```python
from build123d import *

# Parameters (mm, degrees)
EXTRUDE_1_DEPTH     = 20
SKETCH_2_R          = 4
CUT_EXTRUDE_1_DEPTH = 20


with BuildPart() as part:
    # 草图1 → 凸台-拉伸1 (new body)
    with BuildSketch(Plane.XY):
        with BuildLine():
            Line((0, -15), (350, -15))
            ThreePointArc((350, -15), (365, 0), (350, 15))
            Line((350, 15), (0, 15))
            ThreePointArc((0, 15), (-15, 0), (0, -15))
        make_face()
    extrude(amount=EXTRUDE_1_DEPTH)

    # 草图2 → 切除-拉伸1 (cut)
    with BuildSketch(Plane.XY):
        Circle(SKETCH_2_R)
        with Locations((350, 0)):
            Circle(SKETCH_2_R)
    extrude(amount=CUT_EXTRUDE_1_DEPTH, mode=Mode.SUBTRACT)


solid = part.part
```
Verification items for the finished model (mm, model axes). Round coordinates to 2 decimals unless told otherwise and drop trailing zeros. Write each loop counter-clockwise with the first axis right and the second up, starting at its lowest first coordinate (ties: lowest second). Pieces come first, ordered by that corner, then holes. Notation, with made-up numbers: (12.5, 76) -> (29.5, 76) arc R13 ccw to (29.5, 94) -> close; hole circle Ø8 at (52, -13.75). An arc over 180 degrees is marked (long way). Write each question's results on one line, items separated by ' | '. Start each with the question number.
1. Depth check by flat-ended pin: P1, Ø8, axis at y = -9, z = 17, coming from the +X side; P2, Ø1, axis at y = -8, z = 5.5, coming from the -X side; P3, Ø8, axis at y = 10, z = 6.5, coming from the +X side; P4, Ø10, axis at x = 308, y = -10.5, coming from the -Z side. Enter the tip coordinate at first touch or a pass-through.
2. Material ranges on probe 1 along Y at (x, z) = (0, 7.75); probe 2 along X at (y, z) = (13, 16); probe 3 along X at (y, z) = (6, 15), recorded low to high. Write a range as from..to.
3. Cross-section at B-B (z = 7.75). Enter the section's corners in (x, y).
4. Cross-section at A-A (y = 0). Enter the section's corners in (x, z).
5. Draft check along X on faces 1 (the cylindrical face through (-0.867, -3.905, 9.86)), 2 (the cylindrical face through (-15, 0, 10)), 3 (the cylindrical face through (365, 0, 10)). Enter one of: +X half, -X half, draft (parallel to the pull), parting line (faces both ways), or undercut.
Solutions:
1) P1: stops at x = 364.14 | P2: stops at x = -12.99 | P3: stops at x = 363.75 | P4: stops at z = 0
2) probe 1: y = -15..-4, 4..15 | probe 2: x = -7.48..357.48 | probe 3: x = -13.75..363.75
3) outline: (0, -15) -> (350, -15) arc R15 ccw to (350, 15) -> (0, 15) arc R15 ccw to start; hole circle Ø8 at (0, 0); hole circle Ø8 at (350, 0)
4) outline: (-15, 0) -> (-4, 0) -> (-4, 20) -> (-15, 20) -> close; (4, 0) -> (346, 0) -> (346, 20) -> (4, 20) -> close; (354, 0) -> (365, 0) -> (365, 20) -> (354, 20) -> close
5) face 1: undercut | face 2: -X half | face 3: +X half
